Source: CAD feature listing. Evaluate the final solid. Frame: model axes, mm. A direction names the side the tool comes from. Round coordinates to 2 decimals unless told otherwise and drop trailing zeros. Order: outer loops, then holes, each group sorted by start corner. A loop starts at its lowest first (then second) coordinate and runs counter-clockwise, first axis right, second up. Notation, with made-up numbers: (-24.75, -16) - (-2.75, -16) arc R20 cw to (-2.75, 17) - close; hole circle Ø3 at (31, -19). An arc over 180 degrees is marked (long way). Return JSON: item names as keys, results as strings. Group by question number.
1) Contact query for flat-ended pins moving along their axis: P1, Ø1, axis at x = 28.5, y = -41.5, coming from the +Z side; P2, Ø25, axis at x = -1, y = -33.5, coming from the +Z side; P3, Ø12, axis at y = -13.5, z = 14.5, coming from the -X side. Output: stop coordinate, or through.
2) Section A-A, the plane z = -39. Return loops of the section in (x, y).
3) Mould query, pull axis X, two halves, no side actions, for faces 5 (the flat face through (-10, -40, 45)), 6 (the flat face through (-10, -95, -10)), 7 (the cylindrical face through (35.72, -85.49, -11.98)), 8 (the cylindrical face through (48, -60, -25)). Classes: pulls with the +X half, pulls with the -X half, needs draft (parallel to the pull), parting line crosses it, or undercut.
4) Access query for faces 1 (the flat face through (-13, -37, 40)), 2 (the cylindrical face through (13.09, -97.54, -19.58)), 3 (the cylindrical face through (-15.42, -64.406, 47.535)), 4 (the flat face through (45, -40, -10)). Directions: +Z, -Z, +X, -X, +Y, -Y. A direction counts if a zero-diameter tool reaches every point of the face in a straight line with its end or side. Return the directions, or none.
5) Section C-C, the plane x = -10. Return loops of the section in (y, z).
6) Ray query, line 1 (Z direction, x = 8, y = -19.5); line 2 (Y direction, x = 22, z = -37.5). Return the intervals inside material, ascending. Write a range as from..to.
7) Section B-B, the plane y = -40. Return loops of the section in (x, z), plus the area to 3 significant figures.
8) Section D-D, the plane z = 32.5. Return loops of the section in (x, y), plus the area to 3 significant figures.
```python
from build123d import *

# Parameters (mm, degrees)
F0_W     = 100
F0_H     = 100
F1_DEPTH = 100
F2_R     = 25
F3_T     = -10
F4_R     = 25
F5_DEPTH = 5
F6_R     = 25
F7_DEPTH = 5
F8_R     = 25
F9_DEPTH = 5


with BuildPart() as f1:
    # F0 (on Front) → F1 (new body)
    with BuildSketch(Plane.XZ):
        Rectangle(F0_W, F0_H)
    extrude(amount=F1_DEPTH)

    # F2
    f2_edges = [f1.edges().sort_by_distance(p)[0] for p in [
        (0, -100, 50),
        (50, -50, 50),
        (50, -100, 0),
    ]]
    fillet(f2_edges, radius=F2_R)

    # F3
    f3_openings = [f1.faces().sort_by_distance(p)[0] for p in [
        (-50, -49.396169, -0.603831),
        (-0.603831, 0, -0.603831),
        (-0.603831, -49.396169, -50),
    ]]
    offset(amount=F3_T, openings=f3_openings)

    # F4 (on face) → F5 (cut)
    with BuildSketch(Plane.XZ.offset(100)):
        with Locations((-10, -10)):
            Circle(F4_R)
    extrude(amount=-F5_DEPTH, mode=Mode.SUBTRACT)

    # F6 (on face) → F7 (cut)
    with BuildSketch(Plane.YZ.offset(50)):
        with Locations((-40, -10)):
            Circle(F6_R)
    extrude(amount=-F7_DEPTH, mode=Mode.SUBTRACT)

    # F8 (on face) → F9 (cut)
    with BuildSketch(Plane.XY.offset(50)):
        with Locations((-10, -40)):
            Circle(F8_R)
    extrude(amount=-F9_DEPTH, mode=Mode.SUBTRACT)


solid = f1.part
```
Geometry check:
{
 "1": {"P1": "z = 49.82", "P2": "z = 45", "P3": "x = 40"},
 "2": {"outline": "(-50, -100) - (25, -100) arc R25 ccw to (50, -75) - (50, 0) - (40, 0) - (40, -75) arc R15 cw to (25, -90) - (-50, -90) - close"},
 "3": {"face 5": "undercut", "face 6": "undercut", "face 7": "pulls with the -X half", "face 8": "needs draft"},
 "4": {"face 1": "-Z, -X, +Y", "face 2": "-Y", "face 3": "+Z", "face 4": "+X"},
 "5": {"outline": "(-100, -50) - (-90, -50) - (-90, 25) arc R15 cw to (-75, 40) - (0, 40) - (0, 50) - (-15, 50) - (-15, 45) - (-65, 45) - (-65, 50) - (-75, 50) arc R25 ccw to (-100, 25) - (-100, 15) - (-95, 15) - (-95, -35) - (-100, -35) - close"},
 "6": {"line 1": "40..50", "line 2": "-100..-90"},
 "7": {"outline": "(-50, 40) - (25, 40) arc R15 cw to (40, 25) - (40, -50) - (50, -50) - (50, -35) - (45, -35) - (45, 15) - (50, 15) - (50, 25) arc R25 ccw to (25, 50) - (15, 50) - (15, 45) - (-35, 45) - (-35, 50) - (-50, 50) - close", "area": "1,310 mm2"},
 "8": {"outline": "(-50, -98.85) - (25, -98.85) arc R23.85 ccw to (48.85, -75) - (48.85, 0) - (37.99, 0) - (37.99, -75) arc R12.99 cw to (25, -87.99) - (-50, -87.99) - close", "area": "1,940 mm2"}
}
